```python
from build123d import *

# Parameters (mm, degrees)
SKETCH1_W           = 60
SKETCH1_H           = 15
BOSS_EXTRUDE1_DEPTH = 13
SKETCH4_W           = 5
SKETCH4_H           = 15
BOSS_EXTRUDE2_DEPTH = 4
SKETCH2_W           = 50
SKETCH2_H           = 5
CUT_EXTRUDE1_DEPTH  = 10


with BuildPart() as part:
    # Sketch1 → Boss-Extrude1 (new body)
    with BuildSketch(Plane(origin=(0, 0, 0), x_dir=(1, 0, 0), z_dir=(0, 1, 0))):
        Rectangle(SKETCH1_W, SKETCH1_H)
    extrude(amount=BOSS_EXTRUDE1_DEPTH)

    # Sketch4 → Boss-Extrude2 (add)
    with BuildSketch(Plane(origin=(0, 0, 0), x_dir=(-1, 0, 0), z_dir=(0, -1, 0))):
        with Locations((27.5, 0)):
            Rectangle(SKETCH4_W, SKETCH4_H)
    boss_extrude2 = extrude(amount=BOSS_EXTRUDE2_DEPTH)

    # Mirror1: Boss-Extrude2 across plane
    add(boss_extrude2.mirror(Plane(origin=(0, 0, 0), x_dir=(0, 0, 1), z_dir=(1, 0, 0))))

    # Sketch2 → Cut-Extrude1 (cut)
    with BuildSketch(Plane(origin=(0, 13, 0), x_dir=(1, 0, 0), z_dir=(0, 1, 0))):
        Rectangle(SKETCH2_W, SKETCH2_H)
    extrude(amount=-CUT_EXTRUDE1_DEPTH, mode=Mode.SUBTRACT)


solid = part.part
```
The listing builds one solid part. Answer for the finished solid, in the listing's coordinates (mm). A direction names the side the tool comes from. Give positions to 0.01 mm unless a question says otherwise; leave off trailing zeros. Order: outer loops, then holes, each group sorted by start corner. A loop starts at its lowest first (then second) coordinate and runs counter-clockwise, first axis right, second up. Notation, with made-up numbers: (35, 3) -> (85, 3) arc R16 cw to (85, 15) -> close; hole circle Ø1 at (76.5, 38.5). An arc over 180 degrees is marked (long way). Write each question's results on one line, items separated by ' | '.
Q1. Which of the six approach directions +Z, -Z, +X, -X, +Y, -Y give full straight-line access (tool end or side, diameter ignored) to faces 1 (the face through (27, -4, 0)), 2 (the face through (25, 8, 0)), 3 (the face through (-25, -2, 0))?
Checked values:
face 1: +Z, -Z, +X, -X, -Y | face 2: +Y | face 3: +Z, -Z, -Y
Q2. Determine the mould class of faces 4 (the face through (0, 8, -2.5)), 5 (the face through (30, 5, 0)), 6 (the face through (0, 7, 7.5)) for opening direction Z: pulls with the +Z half, pulls with the -Z half, needs draft (parallel to the pull), parting line crosses it, or undercut.
Checked values:
face 4: undercut | face 5: needs draft | face 6: pulls with the +Z half
Q3. The part is cut by section B-B, the plane z = 0.5. Give the vertices of the cut face in (x, y).
Checked values:
outline: (-30, -4) -> (-25, -4) -> (-25, 0) -> (25, 0) -> (25, -4) -> (30, -4) -> (30, 13) -> (25, 13) -> (25, 3) -> (-25, 3) -> (-25, 13) -> (-30, 13) -> close
Q4. The part is cut by section D-D, the plane x = -15. Give the vertices of the cut face in (y, z).
Checked values:
outline: (0, -7.5) -> (13, -7.5) -> (13, -2.5) -> (3, -2.5) -> (3, 2.5) -> (13, 2.5) -> (13, 7.5) -> (0, 7.5) -> close
Q5. Each of these flat-tipped pins is pushed along its axis until it touches: P1, Ø5, axis at x = 5.5, z = -4, coming from the -Y side; P2, Ø5.5, axis at x = -1.5, z = 0, coming from the +Y side. Where does it stop, or does it pass through?
Checked values:
P1: stops at y = 0 | P2: stops at y = 13
Q6. Straight lines are drawn through the part: probe 1 along Z at (x, y) = (-21, 3.75); probe 2 along X at (y, z) = (3.5, -2); probe 3 along Y at (x, z) = (-10, 5.5). For each, find the intervals that lie inside material, in ascending order. Write a range as from..to.
Checked values:
probe 1: z = -7.5..-2.5, 2.5..7.5 | probe 2: x = -30..-25, 25..30 | probe 3: y = 0..13
Q7. The part is cut by section C-C, the plane y = -2.5. Give the vertices of the cut face in (x, z).
Checked values:
outline: (-30, -7.5) -> (-25, -7.5) -> (-25, 7.5) -> (-30, 7.5) -> close; (25, -7.5) -> (30, -7.5) -> (30, 7.5) -> (25, 7.5) -> close
Q8. The part is cut by section A-A, the plane y = 4.5. Give the vertices of the cut face in (x, z), and give its area (3 significant figures).
Checked values:
outline: (-30, -7.5) -> (30, -7.5) -> (30, 7.5) -> (-30, 7.5) -> close; hole (-25, -2.5) -> (25, -2.5) -> (25, 2.5) -> (-25, 2.5) -> close | area: 650 mm^2
